Part model, mm, in its own coordinate system. A direction names the side the tool comes from. Coordinates: 2 decimals unless noted, no trailing zeros. Loops run counter-clockwise (first coordinate to the right, second up) from the corner with the lowest first, then second, coordinate; pieces in that order, holes last. Notation, with made-up numbers: M 88,10.5 L 131,10.5 A11 cw 131,27.5 Z; hole C 73.5,8 d6. An arc over 180 degrees is marked long. Answer as a JSON object with one key per item and string values. Group by question number.
1. Saw through at C-C on z = -0.75. Write the cut outline in (x, y) (3 decimals).
2. Saw through at B-B on x = -5. Write the cut outline in (y, z) (3 decimals).
3. Mould opens along Y. For faces 1 (the face through (-5.158, -2.465, -3.955)), 2 (the face through (-6, 8.175, -11)), 3 (the face through (-4, 3.175, -13)), 4 (the face through (-4.42, -5, 1.54)) say: released by +Y, released by -Y, zero draft, split by the parting line, or undercut.
4. Saw through at D-D on y = 1. Write the cut outline in (x, z).
5. Drop flat-ended pins along their axis: pin 1 Ø1.6 at (y, z) = (10, -11) entering from +X; pin 2 Ø8 at (x, y) = (6.5, -2.5) entering from +Z; pin 3 Ø2.5 at (x, z) = (-4, -8.5) entering from -Y. Give the stop position or say it passes through.
6. Saw through at A-A on y = 11. Write the cut outline in (x, z), then the cut area to 3 significant figures.
7. Drill centre lines: L1, parallel to Y at x = -2, z = -14.5 (3 decimals); L2, parallel to X at y = 5.75, z = 0; L3, parallel to Y at x = -5.75, z = 1 (3 decimals). Where is each one in solid material? Low to high.
8. 3-axis set-ups, long thin cutter, end or side, ignore diameter. For faces 5 (the face through (0, 2, -11)), 6 (the face through (0, 9, -6)), 7 (the face through (-0.59, -6.97, 4.46)), 8 (the face through (-7.407, 8.598, 1.306)): which of +Z, -Z, +X, -X, +Y, -Y reach the whole face in a straight line?
from build123d import *

# Parameters (mm, degrees)
SKETCH1_R           = 9
BOSS_EXTRUDE1_DEPTH = 3.175
BOSS_EXTRUDE2_DEPTH = 11
SKETCH4_R           = 6.5
BOSS_EXTRUDE3_DEPTH = 5
SKETCH5_R           = 4.5
BOSS_EXTRUDE4_DEPTH = 4
BOSS_EXTRUDE5_DEPTH = 3.175
BOSS_EXTRUDE6_DEPTH = 3.175


with BuildPart() as part:
    # Sketch1 → Boss-Extrude1 (new body)
    with BuildSketch(Plane(origin=(0, 0, 0), x_dir=(1, 0, 0), z_dir=(0, 1, 0))):
        Circle(SKETCH1_R)
    extrude(amount=BOSS_EXTRUDE1_DEPTH)

    # Sketch3 → Boss-Extrude2 (add)
    with BuildSketch(Plane(origin=(0, 3.175, 0), x_dir=(1, 0, 0), z_dir=(0, 1, 0))):
        with BuildLine():
            Line((-8.863269777, -1.562833599), (-5.908846518, -1.041889066))
            ThreePointArc((-5.908846518, -1.041889066), (0, 6), (5.908846518, -1.041889066))
            Line((5.908846518, -1.041889066), (8.863269777, -1.562833599))
            ThreePointArc((8.863269777, -1.562833599), (0, 9), (-8.863269777, -1.562833599))
        make_face()
    extrude(amount=BOSS_EXTRUDE2_DEPTH)

    # Sketch4 → Boss-Extrude3 (add)
    with BuildSketch(Plane.XZ):
        Circle(SKETCH4_R)
    extrude(amount=BOSS_EXTRUDE3_DEPTH)

    # Sketch5 → Boss-Extrude4 (add)
    with BuildSketch(Plane.XZ.offset(5)):
        Circle(SKETCH5_R)
    extrude(amount=BOSS_EXTRUDE4_DEPTH)

    # Sketch6 → Boss-Extrude5 (add)
    with BuildSketch(Plane(origin=(0, 0, 0), x_dir=(1, 0, 0), z_dir=(0, 1, 0))):
        with BuildLine():
            Line((-9, 0), (-9, 13))
            ThreePointArc((-9, 13), (-4.5, 17.5), (0, 13))
            Line((0, 13), (0, 9))
            ThreePointArc((0, 9), (-6.363961031, 6.363961031), (-9, 0))
        make_face()
    extrude(amount=BOSS_EXTRUDE5_DEPTH)

    # Sketch7 → Boss-Extrude6 (add)
    with BuildSketch(Plane(origin=(0, 8.174999906, 0), x_dir=(1, 0, 0), z_dir=(0, 1, 0))):
        with BuildLine():
            Line((0, 9), (0, 13))
            ThreePointArc((0, 13), (-4.5, 17.5), (-9, 13))
            Line((-9, 13), (-9, 0))
            ThreePointArc((-9, 0), (-6.363961031, 6.363961031), (0, 9))
        make_face()
    extrude(amount=BOSS_EXTRUDE6_DEPTH)


solid = part.part
Outcome:
{
 "1": {"outline": "M -9,0 L -6.457,0 L -6.457,-5 L -4.437,-5 L -4.437,-9 L 4.437,-9 L 4.437,-5 L 6.457,-5 L 6.457,0 L 8.969,0 L 8.969,14.175 L 5.953,14.175 L 5.953,3.175 L -5.953,3.175 L -5.953,14.175 L -8.969,14.175 L -8.969,11.35 L -9,11.35 L -9,8.175 L -8.969,8.175 L -8.969,3.175 L -9,3.175 Z"},
 "2": {"outline": "M -5,-4.153 L 0,-4.153 L 0,-17.472 L 3.175,-17.472 L 3.175,-7.483 L 8.175,-7.483 L 8.175,-17.472 L 11.35,-17.472 L 11.35,-7.483 L 14.175,-7.483 L 14.175,-3.317 L 3.175,-3.317 L 3.175,7.483 L 0,7.483 L 0,4.153 L -5,4.153 Z"},
 "3": {"face 1": "zero draft", "face 2": "undercut", "face 3": "undercut", "face 4": "released by -Y"},
 "4": {"outline": "M -9,-13 A4.5 ccw 0,-13 L 0,-9 A9 ccw long -9,0 Z"},
 "5": {"pin 1": "stops at x = 0", "pin 2": "stops at z = 8.34", "pin 3": "stops at y = 0"},
 "6": {"outline": "M -9,-13 A4.5 ccw 0,-13 L 0,-9 A9 ccw 8.86,1.56 L 5.91,1.04 A6 cw long -5.91,1.04 L -8.86,1.56 A9 ccw -9,0 Z", "area": "164 mm²"},
 "7": {"L1": "y = 0 to 3.175, 8.175 to 11.35", "L2": "x = -9 to -6, 6 to 9", "L3": "y = -5 to 3.175"},
 "8": {"face 5": "-Z, +X, +Y, -Y", "face 6": "+Y", "face 7": "-Y", "face 8": "+Z, +Y"}
}
